Geometry: see drawing. Coordinates: mm, zero at the bounding-box minimum. Give positions to 0.01 mm unless a question says otherwise; leave off trailing zeros. Loops run counter-clockwise (first coordinate to the right, second up) from the corner with the lowest first, then second, coordinate; pieces in that order, holes last. Notation, with made-up numbers: (-3.5, 20.5) -> (10.5, 20.5) arc R26 ccw to (10.5, 53.5) -> close; hole circle Ø4 at (46, -38.75). An arc over 180 degrees is marked (long way). Answer in a Markdown table with one row per item. Add a question column.
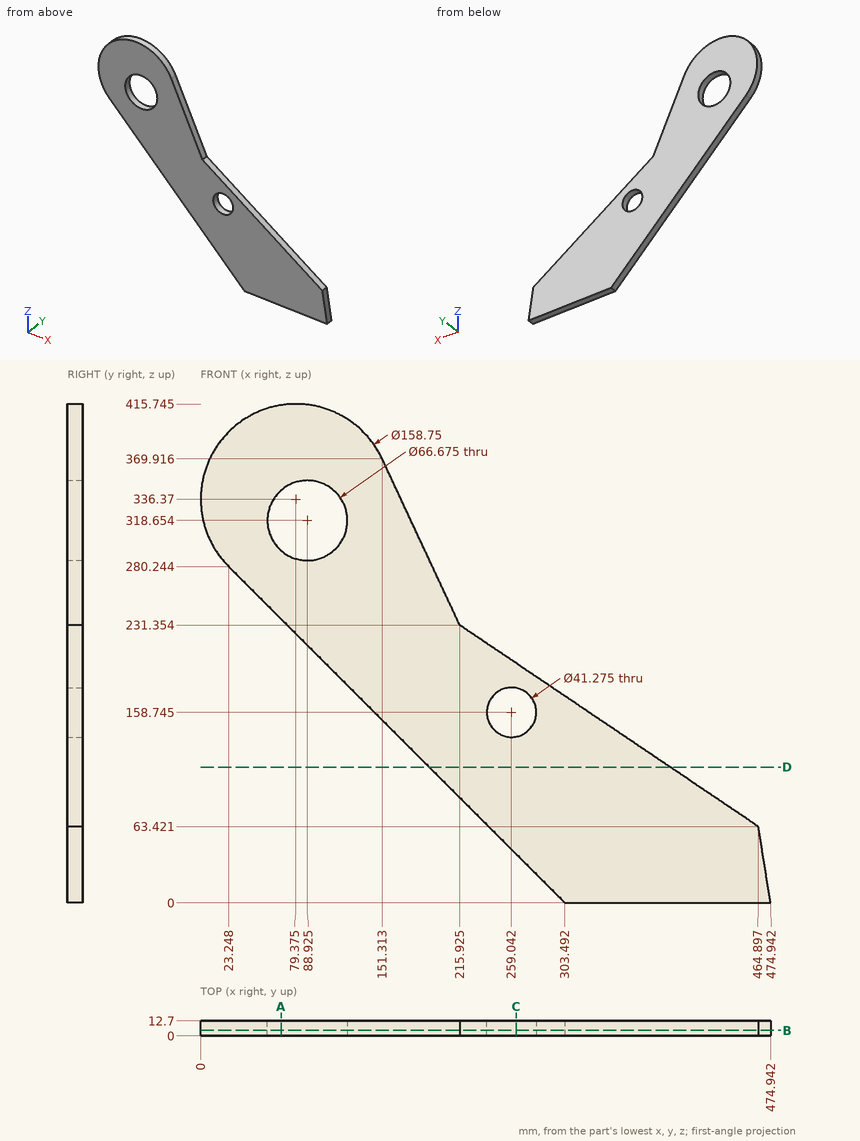
1) Material intervals for line 1 along X through (y, z) = (4.25, 142.5) (1 decimal); line 2 along Z through (x, y) = (257, 5.75); line 3 along Z through (x, y) = (86, 2) (1 decimal), sorted ascending.
2) Section A-A on x = 67. Output: boundary loops of the cut face in (y, z) (1 decimal).
3) Section B-B on y = 4.75. State how many separate pieces and enclosed holes the cut face has, and give its area (3 significant figures).
4) Section D-D on z = 113. Output: boundary loops of the cut face in (x, y), and give its area (3 significant figures).
5) Pin query (flat end, axial travel): pin 1 (6 mm diameter, centred on y = 2, z = 329.5, fed in from +X); pin 2 (2 mm diameter, centred on y = 6.5, z = 296.5, fed in from -X); pin 3 (4 mm diameter, centred on y = 6, z = 146.5, fed in from -X). Return the tip coordinate at first contact, or that it passes through.
6) Section C-C on x = 263. Output: boundary loops of the cut face in (y, z).
Working result:
| question | item | result |
|---|---|---|
| 1 | line 1 | x = 161 to 246.3, 271.8 to 347.7 |
| 1 | line 2 | z = 46.49 to 138.21, 179.28 to 203.65 |
| 1 | line 3 | z = 217.5 to 285.4, 351.9 to 415.5 |
| 2 | outline | (0, 236.5) -> (12.7, 236.5) -> (12.7, 293.5) -> (0, 293.5) -> close; (0, 343.8) -> (12.7, 343.8) -> (12.7, 414.8) -> (0, 414.8) -> close |
| 3 | separate pieces | 1 |
| 3 | enclosed holes | 2 |
| 3 | area | 66,000 mm2 |
| 4 | outline | (190.49, 0) -> (391.39, 0) -> (391.39, 12.7) -> (190.49, 12.7) -> close |
| 4 | area | 2,550 mm2 |
| 5 | pin 1 | stops at x = 171.56 |
| 5 | pin 2 | stops at x = 10.17 |
| 5 | pin 3 | stops at x = 154.99 |
| 6 | outline | (0, 40.49) -> (12.7, 40.49) -> (12.7, 138.49) -> (0, 138.49) -> close; (0, 179) -> (12.7, 179) -> (12.7, 199.6) -> (0, 199.6) -> close |
